```python
from build123d import *

# Parameters (mm, degrees)
EXTRUDE_1_DEPTH     = 50
SKETCH_2_W          = 35
SKETCH_2_H          = 35
CUT_EXTRUDE_1_DEPTH = 116
FILLET_1_R          = 15
SKETCH_3_R          = 10
CUT_EXTRUDE_2_DEPTH = 10
FILLET_2_R          = 20


with BuildPart() as part:
    # 스케치1 → 보스-돌출1 (new body)
    with BuildSketch(Plane(origin=(0, 0, 0), x_dir=(0, 0, -1), z_dir=(1, 0, 0))):
        Polygon((0, 0), (40, 0), (40, 35), (110, 35), (110, -10), (0, -10), align=None)
    extrude(amount=EXTRUDE_1_DEPTH)

    # 스케치2 → 컷-돌출1 (cut)
    with BuildSketch(Plane.XY.offset(-40)):
        with Locations((32.5, 17.5)):
            Rectangle(SKETCH_2_W, SKETCH_2_H)
    extrude(amount=-CUT_EXTRUDE_1_DEPTH, mode=Mode.SUBTRACT)

    # 필렛1
    fillet_1_edges = [part.edges().sort_by_distance(p)[0] for p in [
        (7.5, 35, -40),
        (7.5, 35, -110),
    ]]
    fillet(fillet_1_edges, radius=FILLET_1_R)

    # 스케치3 → 컷-돌출2 (cut)
    with BuildSketch(Plane(origin=(0, 0, 0), x_dir=(1, 0, 0), z_dir=(0, 1, 0))):
        with Locations((26.5, 26.5)):
            Circle(SKETCH_3_R)
    extrude(amount=-CUT_EXTRUDE_2_DEPTH, mode=Mode.SUBTRACT)

    # 필렛2
    fillet_2_edges = [part.edges().sort_by_distance(p)[0] for p in [
        (50, -5, 0),
    ]]
    fillet(fillet_2_edges, radius=FILLET_2_R)


solid = part.part
```
Verification items for the finished model (mm, model axes). A direction names the side the tool comes from. Give positions to 0.01 mm unless a question says otherwise; leave off trailing zeros. Order: outer loops, then holes, each group sorted by start corner. A loop starts at its lowest first (then second) coordinate and runs counter-clockwise, first axis right, second up. Notation, with made-up numbers: (9.25, 29.5) - (47.25, 29.5) arc R21 ccw to (47.25, 49.5) - close; hole circle Ø8 at (30, -39.75). An arc over 180 degrees is marked (long way). Answer as CSV lines item,"result". Start each with the question number.
Item 1: Mould release check, pull along X, two halves, no side actions. Record for faces 4 (the face through (43.986, -4.93, -5.703)), 5 (the face through (36.04, -4.93, -29.5)), 6 (the face through (0, 13, -68)), 7 (the face through (25, -10, -56)): released by +X, released by -X, zero draft, split by the parting line, or undercut.
Item 2: Gauge pin test, flat ends, axial feed: pin 1 (3 mm diameter, centred on y = 2, z = -22, fed in from +X); pin 2 (7.5 mm diameter, centred on x = 5, y = 14.5, fed in from +Z); pin 3 (2 mm diameter, centred on x = 23.5, z = -88, fed in from +Y); pin 4 (8 mm diameter, centred on y = 18.5, z = -82, fed in from +X). Record the tip position at first contact, or that the pin passes through.
Item 3: Access from +Z, -Z, +X, -X, +Y, -Y to the whole of each face (thin tool, end or side, straight path). Record for faces 1 (the face through (15, 17, -75)), 2 (the face through (50, -5, -66)), 3 (the face through (7, 10, -40)).
Item 4: Section check D-D, the plane z = -91. Record the boundary of the cut face in (x, y), plus the area to 4 significant figures.
Item 5: Material ranges on L1, parallel to Z at x = 26.5, y = -2.5; L2, parallel to X at y = -6, z = -26.5; L3, parallel to X at y = 10.5, z = -45, recorded low to high.
Item 6: Section check C-C, the plane x = 3. Record the boundary of the cut face in (y, z), plus the area to 3 significant figures.
Item 7: Section check B-B, the plane z = -26.5. Record the boundary of the cut face in (x, y).
Item 8: Section check A-A, the plane x = 26.5. Record the boundary of the cut face in (y, z), plus the area to 3 significant figures.
Filled in:
1,face 4,"released by +X"
1,face 5,"undercut"
1,face 6,"released by -X"
1,face 7,"zero draft"
2,pin 1,"through"
2,pin 2,"z = -40"
2,pin 3,"y = 0"
2,pin 4,"x = 15"
3,face 1,"+Z, -Z, +X, +Y"
3,face 2,"+Z, -Z, +X, +Y, -Y"
3,face 3,"+Z, +X, -X, +Y"
4,outline,"(0, -10) - (50, -10) - (50, 0) - (15, 0) - (15, 35) - (0, 35) - close"
4,area,"1,025 mm^2"
5,L1,"-110 to -36.5, -16.5 to 0"
5,L2,"0 to 16.5, 36.5 to 50"
5,L3,"0 to 15"
6,outline,"(-10, -110) - (20, -110) arc R15 ccw to (35, -95) - (35, -55) arc R15 ccw to (20, -40) - (0, -40) - (0, 0) - (-10, 0) - close"
6,area,"3,450 mm^2"
7,outline,"(0, -10) - (16.5, -10) - (16.5, 0) - (0, 0) - close; (36.5, -10) - (50, -10) - (50, 0) - (36.5, 0) - close"
8,outline,"(-10, -110) - (0, -110) - (0, -36.5) - (-10, -36.5) - close; (-10, -16.5) - (0, -16.5) - (0, 0) - (-10, 0) - close"
8,area,"900 mm^2"
